Source: CAD feature listing. Evaluate the final solid. Frame: model axes, mm. Round coordinates to 2 decimals unless told otherwise and drop trailing zeros. Order: outer loops, then holes, each group sorted by start corner. A loop starts at its lowest first (then second) coordinate and runs counter-clockwise, first axis right, second up. Notation, with made-up numbers: M 39,41 L 87,41 A31 cw 87,74 Z; hole C -0.5,59.5 d10. An arc over 180 degrees is marked long. Use one line per item in the form item = value. Start each with the question number.
Q1. Section B-B (z = 1). Return the cut outline in (x, y).
Q2. Section A-A (x = 5.5). Return the cut outline in (y, z).
Q3. Material intervals for probe 1 along Y at (x, z) = (-10, 63); probe 2 along Y at (x, z) = (35.5, 28.5); probe 3 along Z at (x, y) = (-17, -130), sorted ascending.
Q4. Section C-C (z = 74.5). Return the cut outline in (x, y), plus the area to 3 significant figures.
Q5. Contact query for flat-ended pins moving along their axis: pin 1 (4 mm diameter, centred on x = -12.5, z = 55, fed in from -Y); pin 2 (10 mm diameter, centred on y = -135.5, z = -10.5, fed in from +X); pin 3 (5 mm diameter, centred on x = -16.5, y = -105, fed in from +Z). Output: stop coordinate, or through.
from build123d import *

# Parameters (mm, degrees)
F0_W     = 100
F0_H     = 140
F1_DEPTH = 300
F4_DEPTH = 140.001
F5_DEPTH = 100.001
F6_ANGLE = 20
F7_ANGLE = 20
F8_W     = 212.240686353
F8_H     = 198.875214911
F9_DEPTH = 142


with BuildPart() as f1:
    # F0 (on Front) → F1 (new body)
    with BuildSketch(Plane.XZ):
        with Locations((50, 70)):
            Rectangle(F0_W, F0_H)
    extrude(amount=F1_DEPTH)

    # F2 (on face) → F4 (cut, through all)
    with BuildSketch(Plane.XY.offset(140)):
        Polygon((50, -300), (0, 0), (-43.4896158054, -321.4669823647), (163.4580759332, -380.9873461723), (100, 0), align=None)
    extrude(amount=-F4_DEPTH, mode=Mode.SUBTRACT)

    # F3 (on face) → F5 (cut, through all)
    with BuildSketch(Plane.YZ.offset(100)):
        Polygon((-300, 70), (0, 140), (-333.8288962841, 174.1326918269), (-333.8288962841, -23.4987252064), (0, 0), align=None)
    extrude(amount=-F5_DEPTH, mode=Mode.SUBTRACT)


with BuildPart() as f1_1:
    # F6: moved
    add(f1.part.rotate(Axis((100, 0, 70), (0, 0, -1)), F6_ANGLE))


with BuildPart() as f1_2:
    # F7: moved
    add(f1_1.part.rotate(Axis((53.0153689607, 17.1010071663, 140), (0.9396926208, -0.3420201433, 0)), F7_ANGLE))

    # F8 (on Top) → F9 (cut, symmetric)
    with BuildSketch(Plane.XY):
        with Locations((27.6002858933, 24.7314047101)):
            Rectangle(F8_W, F8_H)
    extrude(amount=F9_DEPTH, both=True, mode=Mode.SUBTRACT)


solid = f1_2.part
Results list:
q1.outline = M -28.02,-180.02 L -11.62,-185.99 L 49.82,-74.71 L -7.36,-74.71 Z
q2.outline = M -157.47,22.32 L -152.71,-18.49 L -74.71,-9.67 L -74.71,73.08 Z
q3.probe_1 = -85.5 to -74.71
q3.probe_2 = -103.84 to -74.71
q3.probe_3 = -16.85 to 34.14
q4.outline = M 11.86,-74.71 L 47.4,-87.64 L 54.54,-74.71 Z
q4.area = 276 mm2
q5.pin_1 = -100.97
q5.pin_2 = 18.29
q5.pin_3 = 51.22
